Here's how the part is built. I have some questions about the finished solid (model axes, mm). Give positions to 0.01 mm unless a question says otherwise; leave off trailing zeros. Write each loop counter-clockwise with the first axis right and the second up, starting at its lowest first coordinate (ties: lowest second). Pieces come first, ordered by that corner, then holes. Notation, with made-up numbers: M -11,84.5 L 25,84.5 A18 ccw 25,94.5 Z; hole C 1.5,36 d5. An arc over 180 degrees is marked long. Use one line per item in the form item = value. Start each with the question number.
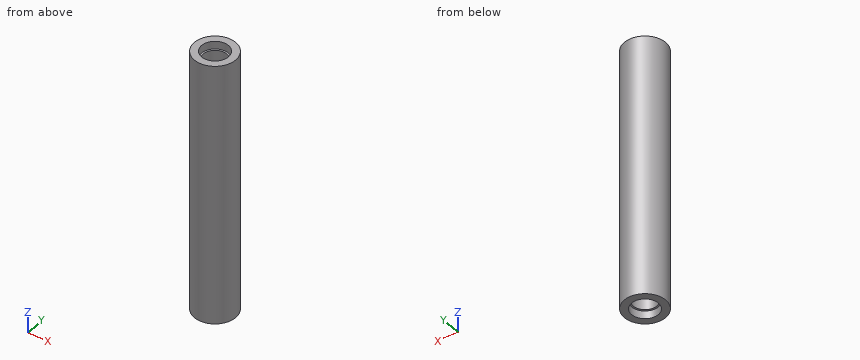
from build123d import *

# Parameters (mm, degrees)
SCHIZZO1_R               = 40
SCHIZZO1_R_2             = 22.5
ESTRUSIONE1_DEPTH        = 252.5
TAGLIO_ESTRUSIONE1_START = -15
SCHIZZO2_R               = 26
SCHIZZO2_R_2             = 22.5
TAGLIO_ESTRUSIONE1_DEPTH = 15
SCHIZZO3_R               = 26
SCHIZZO3_R_2             = 22.5
TAGLIO_ESTRUSIONE2_DEPTH = 15


with BuildPart() as part:
    # Schizzo1 → Estrusione1 (new, symmetric)
    with BuildSketch(Plane.XY):
        Circle(SCHIZZO1_R)
        Circle(SCHIZZO1_R_2, mode=Mode.SUBTRACT)
    extrude(amount=ESTRUSIONE1_DEPTH, both=True)

    # Schizzo2 → Taglio-Estrusione1 (cut)
    with BuildSketch(Plane.XY.offset(252.5).offset(TAGLIO_ESTRUSIONE1_START)):
        Circle(SCHIZZO2_R)
        Circle(SCHIZZO2_R_2, mode=Mode.SUBTRACT)
    extrude(amount=TAGLIO_ESTRUSIONE1_DEPTH, mode=Mode.SUBTRACT)

    # Schizzo3 → Taglio-Estrusione2 (cut)
    with BuildSketch(Plane(origin=(0, 0, -252.5), x_dir=(-1, 0, 0), z_dir=(0, 0, -1))):
        with Locations(Location((0, 0, 0), (0, 0, 180))):
            Circle(SCHIZZO3_R)
        Circle(SCHIZZO3_R_2, mode=Mode.SUBTRACT)
    extrude(amount=-TAGLIO_ESTRUSIONE2_DEPTH, mode=Mode.SUBTRACT)


solid = part.part
1) Will these pins go through, and if not, where does the flat tip stop? P1, Ø1, axis at x = 23.5, z = 49, coming from the +Y side; P2, Ø3, axis at x = -13.5, y = -20, coming from the +Z side; P3, Ø5, axis at x = -29.5, z = 1, coming from the -Y side; P4, Ø1, axis at y = -0.5, z = 137.5, coming from the -X side.
2) Suppose I cut it at A-A, the plane x = 0. List the corners of the cut face in (y, z) for me, and give its area (3 significant figures).
3) Suppose I cut it at D-D, the plane y = -30.5. List the corners of the cut face in (x, z) for me, and give its area (3 significant figures).
4) Please list where these lines run through material, in increasing order: line 1 (Y direction, x = 0, z = 37); line 2 (Y direction, x = 2, z = -3); line 3 (X direction, y = 10, z = -93).
5) Suppose I cut it at C-C, the plane z = -55. List the corners of the cut face in (x, y) for me, and give its area (3 significant figures).
Checks:
q1.P1 = 32.73
q1.P2 = 237.5
q1.P3 = -29.51
q1.P4 = -40
q2.outline = M -40,-252.5 L -26,-252.5 L -26,-237.5 L -22.5,-237.5 L -22.5,237.5 L -26,237.5 L -26,252.5 L -40,252.5 Z; M 22.5,-237.5 L 26,-237.5 L 26,-252.5 L 40,-252.5 L 40,252.5 L 26,252.5 L 26,237.5 L 22.5,237.5 Z
q2.area = 17,500 mm^2
q3.outline = M -25.88,-252.5 L 25.88,-252.5 L 25.88,252.5 L -25.88,252.5 Z
q3.area = 26,100 mm^2
q4.line_1 = -40 to -22.5, 22.5 to 40
q4.line_2 = -39.95 to -22.41, 22.41 to 39.95
q4.line_3 = -38.73 to -20.16, 20.16 to 38.73
q5.outline = C 0,0 d80; hole C 0,0 d45
q5.area = 3,440 mm^2
